Build history of the part. All positions in model axes, mm. A direction names the side the tool comes from. Coordinates: 2 decimals unless noted, no trailing zeros. Loops run counter-clockwise (first coordinate to the right, second up) from the corner with the lowest first, then second, coordinate; pieces in that order, holes last.
Item 1: Flat gauge pins, fed straight in: pin 1 (0.7 mm diameter, centred on x = -7.5, z = 1.5, fed in from +Y); pin 2 (4 mm diameter, centred on y = 4.5, z = -6, fed in from -X); pin 3 (5 mm diameter, centred on y = 21, z = 1.5, fed in from -X). Where does each tip first touch, or does it go through?
Item 2: Mould opens along Z. For faces 6 (the face through (-4.99, 19.55, -5.6)), 7 (the face through (4.66, 6.26, 0.61)), 8 (the face through (5.01, 19.21, 5.65)) say: released by +Z, released by -Z, zero draft, split by the parting line, or undercut.
Item 3: 3-axis set-ups, long thin cutter, end or side, ignore diameter. For faces 1 (the face through (-7, 15.24, 0)), 2 (the face through (0, 15, -8)), 3 (the face through (0, 15.24, 0)), 4 (the face through (0, 12.7, 0)), 5 (the face through (6.668, 18, 0)): which of +Z, -Z, +X, -X, +Y, -Y reach the whole face in a straight line?
Item 4: Cut at C-C (x = 5). List the corners of the cut face in (y, z) (1 decimal), and give its area (3 significant figures).
Item 5: Cut at B-B (z = -0.5). List the corners of the cut face in (x, y).
Item 6: Drill centre lines: line 1 along X through (y, z) = (22.25, 0); line 2 along X through (y, z) = (8, 0); line 3 along Z through (x, y) = (3.75, 2). Where is each one in solid material? Low to high.
Item 7: Cut at A-A (x = 0). List the corners of the cut face in (y, z).
Item 8: Cut at D-D (y = 17.25). List the corners of the cut face in (x, z).
from build123d import *

# Parameters (mm, degrees)
SKETCH1_R               = 8.001
BOSS_EXTRUDE1_DEPTH     = 25.4
SKETCH2_R               = 8.001
SKETCH2_R_2             = 6.35
SKETCH2_R_3             = 4.699
CUT_EXTRUDE1_DEPTH      = 12.7
CUT_EXTRUDE2_DEPTH      = 28.806330251
CUT_EXTRUDE2_DEPTH_BACK = 28.806330251
SKETCH3_W               = 8.255
SKETCH3_H               = 10.16
SKETCH3_W_2             = 1.3335
CUT_EXTRUDE3_DEPTH      = 31.402975072


with BuildPart() as part:
    # Sketch1 → Boss-Extrude1 (new body)
    with BuildSketch(Plane(origin=(0, 0, 0), x_dir=(1, 0, 0), z_dir=(0, 1, 0))):
        with Locations(Location((0, 0, 0), (0, 0, 270))):
            Circle(SKETCH1_R)
    extrude(amount=BOSS_EXTRUDE1_DEPTH)

    # Sketch2 → Cut-Extrude1 (cut)
    # profile 1 of 2: a face of its own
    with BuildSketch(Plane(origin=(0, 0, 0), x_dir=(-1, 0, 0), z_dir=(0, -1, 0))):
        with Locations(Location((0, 0, 0), (0, 0, 90))):
            Circle(SKETCH2_R)
        with Locations(Location((0, 0, 0), (0, 0, 90))):
            Circle(SKETCH2_R_2, mode=Mode.SUBTRACT)
    # profile 2 of 2: a face of its own
    with BuildSketch(Plane(origin=(0, 0, 0), x_dir=(-1, 0, 0), z_dir=(0, -1, 0))):
        with Locations(Location((0, 0, 0), (0, 0, 90))):
            Circle(SKETCH2_R_3)
    extrude(amount=-CUT_EXTRUDE1_DEPTH, mode=Mode.SUBTRACT)

    # Sketch3 → Cut-Extrude2 (cut, two sides: drawn at the far end of the back side and taken through both)
    with BuildSketch(Plane.XY.offset(-CUT_EXTRUDE2_DEPTH_BACK)):
        with Locations((0, 20.32)):
            Rectangle(SKETCH3_W, SKETCH3_H)
        with Locations((-7.33425, 20.32)):
            Rectangle(SKETCH3_W_2, SKETCH3_H)
        with Locations((7.33425, 20.32)):
            Rectangle(SKETCH3_W_2, SKETCH3_H)
    extrude(amount=CUT_EXTRUDE2_DEPTH + CUT_EXTRUDE2_DEPTH_BACK, mode=Mode.SUBTRACT)

    # Sketch4 → Cut-Extrude3 (cut, through all)
    with BuildSketch(Plane(origin=(6.6675, 0, 0), x_dir=(0, 0, -1), z_dir=(1, 0, 0))):
        with BuildLine():
            Line((-4.422719158, 25.4), (0, 25.4))
            Line((0, 25.4), (4.422719158, 25.4))
            Line((4.422719158, 25.4), (4.422719158, 22.819190919))
            ThreePointArc((4.422719158, 22.819190919), (4.646674927, 22.373000761), (4.825752455, 21.906982432))
            Line((4.825752455, 21.906982432), (7.018236237, 15.24))
            Line((7.018236237, 15.24), (6.955993892, 50.8))
            Line((6.955993892, 50.8), (-6.858660717, 50.8))
            Line((-6.858660717, 50.8), (-6.858660717, 15.24))
            Line((-6.858660717, 15.24), (-4.859385257, 21.800802121))
            ThreePointArc((-4.859385257, 21.800802121), (-4.668901855, 22.321937928), (-4.422719158, 22.819190919))
            Line((-4.422719158, 22.819190919), (-4.422719158, 25.4))
        make_face()
        with BuildLine():
            ThreePointArc((1.5875, 20.32), (1.122532015, 21.442532015), (0, 21.9075))
            Line((0, 21.9075), (0, 18.7325))
            ThreePointArc((0, 18.7325), (1.122532015, 19.197467985), (1.5875, 20.32))
        make_face()
        with BuildLine():
            Line((0, 18.7325), (0, 21.9075))
            ThreePointArc((0, 21.9075), (-1.5875, 20.32), (0, 18.7325))
        make_face()
        with BuildLine():
            ThreePointArc((-4.422719158, 22.819190919), (-2.560323235, 24.707612669), (0, 25.4))
            Line((0, 25.4), (-4.422719158, 25.4))
            Line((-4.422719158, 25.4), (-4.422719158, 22.819190919))
        make_face()
        with BuildLine():
            Line((4.422719158, 25.4), (0, 25.4))
            ThreePointArc((0, 25.4), (2.560323235, 24.707612669), (4.422719158, 22.819190919))
            Line((4.422719158, 22.819190919), (4.422719158, 25.4))
        make_face()
    extrude(amount=-CUT_EXTRUDE3_DEPTH, mode=Mode.SUBTRACT)


solid = part.part
Filled sheet:
1. pin 1: stops at y = 15.24
1. pin 2: stops at x = -4.93
1. pin 3: stops at x = -6.67
2. face 6: released by -Z
2. face 7: undercut
2. face 8: released by +Z
3. face 1: +Z, -Z, -X, +Y
3. face 2: +Y, -Y
3. face 3: +Z, -Z, +Y
3. face 4: -Y
3. face 5: +Z, -Z, +X, +Y
4. outline: (0, -3.9) - (12.7, -3.9) - (12.7, -6.2) - (17.6, -6.2) - (21.9, -4.8) arc R5.1 ccw to (21.8, 4.9) - (17.2, 6.2) - (12.7, 6.2) - (12.7, 3.9) - (0, 3.9) - close; hole circle Ø3.2 at (20.3, 0)
4. area: 225 mm2
5. outline: (-7.99, 12.7) - (-6.33, 12.7) - (-6.33, 0) - (-4.67, 0) - (-4.67, 12.7) - (4.67, 12.7) - (4.67, 0) - (6.33, 0) - (6.33, 12.7) - (7.99, 12.7) - (7.99, 15.24) - (6.67, 15.24) - (6.67, 18.81) - (4.13, 18.81) - (4.13, 15.24) - (-4.13, 15.24) - (-4.13, 18.81) - (-6.67, 18.81) - (-6.67, 15.24) - (-7.99, 15.24) - close; (-6.67, 21.83) - (-4.13, 21.83) - (-4.13, 25.38) - (-6.67, 25.38) - close; (4.13, 21.83) - (6.67, 21.83) - (6.67, 25.38) - (4.13, 25.38) - close
6. line 1: x = -6.67 to -4.13, 4.13 to 6.67
6. line 2: x = -6.35 to -4.7, 4.7 to 6.35
6. line 3: z = -5.12 to -2.83, 2.83 to 5.12
7. outline: (0, -6.35) - (12.7, -6.35) - (12.7, -8) - (15.24, -8) - (15.24, 8) - (12.7, 8) - (12.7, 6.35) - (0, 6.35) - (0, 4.7) - (12.7, 4.7) - (12.7, -4.7) - (0, -4.7) - close
8. outline: (-6.67, -4.42) arc R8 ccw to (-4.86, -6.36) - (-4.13, -6.36) - (-4.13, 6.25) - (-5, 6.25) arc R8 ccw to (-6.67, 4.42) - close; (4.13, -6.36) - (4.86, -6.36) arc R8 ccw to (6.67, -4.42) - (6.67, 4.42) arc R8 ccw to (5, 6.25) - (4.13, 6.25) - close
